Here's how the part is built. I have some questions about the finished solid (model axes, mm). Face numbers are marked on the shaded views. A direction names the side the tool comes from. Round coordinates to 2 decimals unless told otherwise and drop trailing zeros. Order: outer loops, then holes, each group sorted by start corner. A loop starts at its lowest first (then second) coordinate and runs counter-clockwise, first axis right, second up. Notation, with made-up numbers: (20, -36.5) - (35, -36.5) arc R11 cw to (35, -23.5) - close; hole circle Ø7 at (6.25, -27.75). An arc over 180 degrees is marked (long way). Answer as a JSON object with one key per item and string values.
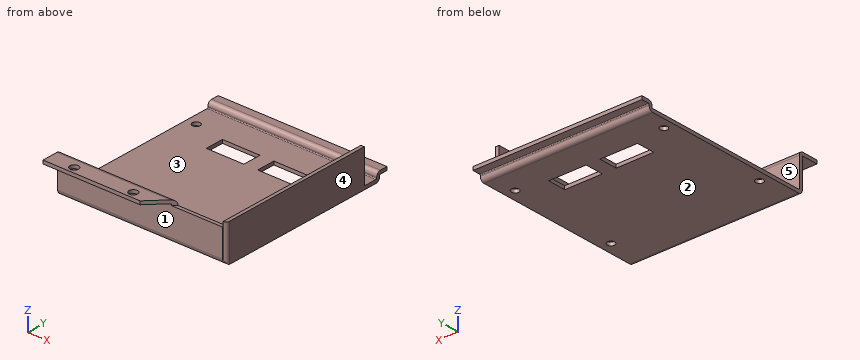
```python
from build123d import *

# Parameters (mm, degrees)
BOSS_EXTRUDE1_DEPTH = 100
SKETCH2_W           = 2.5
SKETCH2_H           = 12.5
CUT_EXTRUDE1_DEPTH  = 21
SKETCH3_W           = 2
SKETCH3_H           = 93.5
BOSS_EXTRUDE2_DEPTH = 20
SKETCH4_R           = 2.5
CUT_EXTRUDE3_DEPTH  = 3
SKETCH5_R           = 2.25
SKETCH5_W           = 22.25
SKETCH5_H           = 10.95
CUT_EXTRUDE4_DEPTH  = 5
FILLET1_R           = 1.8


with BuildPart() as part:
    # Sketch1 → Boss-Extrude1 (new body)
    with BuildSketch(Plane(origin=(0, 0, 0), x_dir=(0, 0, -1), z_dir=(1, 0, 0))):
        with BuildLine():
            Line((0, -2.5), (0, -12))
            Line((0, -12), (2, -12))
            Line((2, -12), (2, -2.5))
            ThreePointArc((2, -2.5), (2.146446609, -2.146446609), (2.5, -2))
            Line((2.5, -2), (19.5, -2))
            ThreePointArc((19.5, -2), (21.267766953, -1.267766953), (22, 0.5))
            Line((22, 0.5), (22, 99.5))
            ThreePointArc((22, 99.5), (21.267766953, 101.267766953), (19.5, 102))
            Line((19.5, 102), (19, 102))
            ThreePointArc((19, 102), (18.646446609, 102.146446609), (18.5, 102.5))
            Line((18.5, 102.5), (18.5, 107))
            Line((18.5, 107), (16.5, 107))
            Line((16.5, 107), (16.5, 102.5))
            ThreePointArc((16.5, 102.5), (17.232233047, 100.732233047), (19, 100))
            Line((19, 100), (19.5, 100))
            ThreePointArc((19.5, 100), (19.853553391, 99.853553391), (20, 99.5))
            Line((20, 99.5), (20, 0.5))
            ThreePointArc((20, 0.5), (19.853553391, 0.146446609), (19.5, 0))
            Line((19.5, 0), (2.5, 0))
            ThreePointArc((2.5, 0), (0.732233047, -0.732233047), (0, -2.5))
        make_face()
    extrude(amount=BOSS_EXTRUDE1_DEPTH)

    # Sketch2 → Cut-Extrude1 (cut, through all)
    with BuildSketch(Plane.XY.offset(-20)):
        with Locations((98.75, -5.75)):
            Rectangle(SKETCH2_W, SKETCH2_H)
    extrude(amount=CUT_EXTRUDE1_DEPTH, mode=Mode.SUBTRACT)

    # Sketch3 → Boss-Extrude2 (add)
    with BuildSketch(Plane.XY.offset(-20)):
        with Locations((99, 44.800510257)):
            Rectangle(SKETCH3_W, SKETCH3_H)
    extrude(amount=BOSS_EXTRUDE2_DEPTH)

    # Sketch4 → Cut-Extrude3 (cut)
    with BuildSketch(Plane.XY):
        with Locations((15, -8)):
            Circle(SKETCH4_R)
        with Locations((50, -8)):
            Circle(SKETCH4_R)
        Polygon((97.5, 0), (69.5, 0), (57.5, -12), (97.5, -12), align=None)
    extrude(amount=-CUT_EXTRUDE3_DEPTH, mode=Mode.SUBTRACT)

    # Sketch5 → Cut-Extrude4 (cut)
    with BuildSketch(Plane.XY.offset(-20)):
        with Locations((5.85, 85.37)):
            Circle(SKETCH5_R)
        with Locations((5.85, 20.37)):
            Circle(SKETCH5_R)
        with Locations((93.85, 20.37)):
            Circle(SKETCH5_R)
        with Locations((93.85, 85.37)):
            Circle(SKETCH5_R)
        with Locations((35.075, 76.945)):
            Rectangle(SKETCH5_W, SKETCH5_H)
        with Locations((65.525, 76.945)):
            Rectangle(SKETCH5_W, SKETCH5_H)
    extrude(amount=-CUT_EXTRUDE4_DEPTH, mode=Mode.SUBTRACT)

    # Fillet1
    fillet1_edges = [part.edges().sort_by_distance(p)[0] for p in [
        (100, -1.949489743, -10),
    ]]
    fillet(fillet1_edges, radius=FILLET1_R)


solid = part.part
```
1. Thinking about a two-plate mould opening in Y: for the marked faces 1, 2 and 3, which applies, pulls with the +Y half, pulls with the -Y half, needs draft (parallel to the pull), parting line crosses it, or undercut?
Responses:
{"face 1": "pulls with the -Y half", "face 2": "needs draft", "face 3": "undercut"}
2. Imagine slicing it at B-B (y = -8). List the corners of the cut face in (x, z) for me, plus the area to 3 significant figures.
Responses:
{"outline": "(0, -2) - (12.5, -2) - (12.5, 0) - (0, 0) - close; (17.5, -2) - (47.5, -2) - (47.5, 0) - (17.5, 0) - close; (52.5, -2) - (61.5, -2) - (61.5, 0) - (52.5, 0) - close", "area": "103 mm2"}
3. Imagine slicing it at A-A (x = 93.85). List the corners of the cut face in (y, z) for me.
Responses:
{"outline": "(-2, -19.5) arc R2.5 ccw to (0.5, -22) - (18.12, -22) - (18.12, -20) - (0.5, -20) arc R0.5 cw to (0, -19.5) - (0, -3) - (-2, -3) - close; (22.62, -22) - (83.12, -22) - (83.12, -20) - (22.62, -20) - close; (87.62, -22) - (99.5, -22) arc R2.5 ccw to (102, -19.5) - (102, -19) arc R0.5 cw to (102.5, -18.5) - (107, -18.5) - (107, -16.5) - (102.5, -16.5) arc R2.5 ccw to (100, -19) - (100, -19.5) arc R0.5 cw to (99.5, -20) - (87.62, -20) - close"}
4. Imagine slicing it at C-C (x = 64). List the corners of the cut face in (y, z) for me, plus the area to 3 significant figures.
Responses:
{"outline": "(-5.5, -2) - (-2.5, -2) arc R0.5 cw to (-2, -2.5) - (-2, -19.5) arc R2.5 ccw to (0.5, -22) - (71.47, -22) - (71.47, -20) - (0.5, -20) arc R0.5 cw to (0, -19.5) - (0, -2.5) arc R2.5 ccw to (-2.5, 0) - (-5.5, 0) - close; (82.42, -22) - (99.5, -22) arc R2.5 ccw to (102, -19.5) - (102, -19) arc R0.5 cw to (102.5, -18.5) - (107, -18.5) - (107, -16.5) - (102.5, -16.5) arc R2.5 ccw to (100, -19) - (100, -19.5) arc R0.5 cw to (99.5, -20) - (82.42, -20) - close", "area": "245 mm2"}
5. For the marked faces 4 and 5, which set-ups out of +Z, -Z, +X, -X, +Y, -Y let a thin tool reach every point of the face, with its end or its side?
Responses:
{"face 4": "+Z, -Z, +X, +Y, -Y", "face 5": "+Z, -X"}
6. If I drill on L1, parallel to Y at x = 15, z = -1.6; L2, parallel to Y at x = 5.85, z = -21.6; L3, parallel to Y at x = 93.85, z = -20.35, over which ranges is the centre line in solid material (lowest first)? Write a range as [from, to].
Responses:
{"L1": "[-12, -10.5], [-5.5, -0.17]", "L2": "[-0.86, 18.12], [22.62, 83.12], [87.62, 100.86]", "L3": "[-1.85, 18.12], [22.62, 83.12], [87.62, 101.85]"}
7. Imagine slicing it at D-D (y = 85.37). List the corners of the cut face in (x, z) for me, plus the area to 3 significant figures.
Responses:
{"outline": "(0, -22) - (3.6, -22) - (3.6, -20) - (0, -20) - close; (8.1, -22) - (91.6, -22) - (91.6, -20) - (8.1, -20) - close; (96.1, -22) - (100, -22) - (100, 0) - (98, 0) - (98, -20) - (96.1, -20) - close", "area": "222 mm2"}
8. For P1, Ø1, axis at x = 69.5, y = 2.5, coming from the +Z side; P2, Ø2, axis at x = 64.5, z = -21.5, coming from the -Y side; P3, Ø5, axis at x = 57.5, y = 104.5, coming from the +Z side, each with a flat end and sliding along its axis, tell me the tip position at first contact or that it passes through.
Responses:
{"P1": "z = -20", "P2": "y = -1.79", "P3": "z = -16.5"}
